from build123d import *

# Parameters (mm, degrees)
BOX021_W               = 30
BOX021_H               = 100
BOX021_DEPTH           = 30
BOX021_PLACEMENT_ANGLE = 45
BOX020_W               = 30
BOX020_H               = 100
BOX020_DEPTH           = 30
BOX020_PLACEMENT_ANGLE = -45
PAD_DEPTH              = 876


with BuildPart() as cube006:
    # Box021 → Box021 (new body)
    with BuildSketch(Plane.XY):
        with Locations((15, 50)):
            Rectangle(BOX021_W, BOX021_H)
    extrude(amount=BOX021_DEPTH)


with BuildPart() as cube006_1:
    # Box021 placement: moved
    add(cube006.part.moved(Location((873, -3, -3))).rotate(Axis((873, -3, -3), (0, 0, 1)), BOX021_PLACEMENT_ANGLE))


with BuildPart() as cube:
    # Box020 → Box020 (new body)
    with BuildSketch(Plane.XY):
        with Locations((15, 50)):
            Rectangle(BOX020_W, BOX020_H)
    extrude(amount=BOX020_DEPTH)


with BuildPart() as cube_1:
    # Box020 placement: moved
    add(cube.part.moved(Location((-24.213203, 18.213203, -3))).rotate(Axis((-24.213203, 18.213203, -3), (0, 0, 1)), BOX020_PLACEMENT_ANGLE))


with BuildPart() as rahmen1:
    # Sketch → Pad (new body)
    with BuildSketch(Plane(origin=(-3, -3, -3), x_dir=(0, 1, 0), z_dir=(1, 0, 0))):
        Polygon((0, 0), (30, 0), (30, 3), (3, 3), (3, 20), (0, 20), align=None)
    extrude(amount=PAD_DEPTH)

    # Cut: cut Cube
    add(cube_1.part, mode=Mode.SUBTRACT)

    # Cut001: cut Cube006
    add(cube006_1.part, mode=Mode.SUBTRACT)


solid = rahmen1.part
Design review of the part built by this model. Coordinates are the model's own, in mm. A direction names the side the tool comes from. Round coordinates to 2 decimals unless told otherwise and drop trailing zeros. Loops run counter-clockwise (first coordinate to the right, second up) from the corner with the lowest first, then second, coordinate; pieces in that order, holes last. Notation, with made-up numbers: (51.5, 38.25) - (96.5, 38.25) arc R31 ccw to (96.5, 71.25) - close; hole circle Ø1 at (30, -31.75). An arc over 180 degrees is marked (long way). One line per item, written item: value. Start each with the question number.
1) To check wall thickness, follow L1, parallel to Z at x = 69, y = 7.5; L2, parallel to X at y = 4.5, z = -1.5. State the ranges of each line that lie inside material, in increasing order. Write a range as from..to.
2) Consider section A-A on x = 237.5. Give the boundary of the cut face in (y, z), then the cut area to 3 significant figures.
3) For faces 1 (the flat face through (429, 0, 8)), 2 (the flat face through (6, 6, -1)), list the 3-axis set-ups (+Z, -Z, +X, -X, +Y, -Y) from which the entire face can be reached by the end or side of a thin tool; tool diameter is ignored.
4) Consider section B-B on y = 8.5. Give the boundary of the cut face in (x, z).
5) Consider section C-C on z = 9.5. Give the boundary of the cut face in (x, y).
6) Insertion check: pin 1 Ø5 at (y, z) = (18.5, 2) entering from +X; pin 2 Ø4 at (x, y) = (434.5, 21) entering from +Z; pin 3 Ø8.5 at (x, z) = (590.5, 7) entering from +Y. Each pin has a flat end and moves straight along its axis. Give the tip position at first contact, or say it passes through.
Reported:
1. L1: z = -3..0
1. L2: x = 4.5..865.5
2. outline: (-3, -3) - (27, -3) - (27, 0) - (0, 0) - (0, 17) - (-3, 17) - close
2. area: 141 mm^2
3. face 1: +Z, +X, -X, +Y
3. face 2: +Z, -Z, -X, +Y
4. outline: (8.5, -3) - (861.5, -3) - (861.5, 0) - (8.5, 0) - close
5. outline: (-3, -3) - (873, -3) - (870, 0) - (0, 0) - close
6. pin 1: stops at x = 853
6. pin 2: stops at z = 0
6. pin 3: stops at y = 0
